Geometry check sheet. Reference: the model listing, model coordinates, mm. Face numbers are marked on the shaded views. A direction names the side the tool comes from. Round coordinates to 2 decimals unless told otherwise and drop trailing zeros. Write each loop counter-clockwise with the first axis right and the second up, starting at its lowest first coordinate (ties: lowest second). Pieces come first, ordered by that corner, then holes. Notation, with made-up numbers: (-7.5, 19.5) -> (25.5, 19.5) arc R22 ccw to (25.5, 46.5) -> close; hole circle Ø2 at (-33.75, 49.25). An arc over 180 degrees is marked (long way). Use a Markdown table: item, result.
```python
from build123d import *

# Parameters (mm, degrees)
BOSS_EXTRUDE1_DEPTH = 12
SKETCH2_R           = 17.5
BOSS_EXTRUDE2_DEPTH = 1
SKETCH3_R           = 0.75
BOSS_EXTRUDE3_DEPTH = 5
FILLET1_R           = 1.5
CUT_EXTRUDE6_REACH  = 67.15
SKETCH6_R           = 2.85
CHAMFER1_SIZE       = 0.5


with BuildPart() as part:
    # Sketch1 → Boss-Extrude1 (new body)
    with BuildSketch(Plane(origin=(0, 0, 0), x_dir=(1, 0, 0), z_dir=(0, 1, 0))):
        with BuildLine():
            Line((-28.55, 22.55), (-28.55, -22.55))
            ThreePointArc((-28.55, -22.55), (-26.792640687, -26.792640687), (-22.55, -28.55))
            Line((-22.55, -28.55), (22.55, -28.55))
            ThreePointArc((22.55, -28.55), (26.792640687, -26.792640687), (28.55, -22.55))
            Line((28.55, -22.55), (28.55, 22.55))
            ThreePointArc((28.55, 22.55), (26.792640687, 26.792640687), (22.55, 28.55))
            Line((22.55, 28.55), (-22.55, 28.55))
            ThreePointArc((-22.55, 28.55), (-26.792640687, 26.792640687), (-28.55, 22.55))
        make_face()
        with BuildLine():
            Line((-22.55, 27.55), (22.55, 27.55))
            ThreePointArc((22.55, 27.55), (26.085533906, 26.085533906), (27.55, 22.55))
            Line((27.55, 22.55), (27.55, -22.55))
            ThreePointArc((27.55, -22.55), (26.085533906, -26.085533906), (22.55, -27.55))
            Line((22.55, -27.55), (-22.55, -27.55))
            ThreePointArc((-22.55, -27.55), (-26.085533906, -26.085533906), (-27.55, -22.55))
            Line((-27.55, -22.55), (-27.55, 22.55))
            ThreePointArc((-27.55, 22.55), (-26.085533906, 26.085533906), (-22.55, 27.55))
        make_face(mode=Mode.SUBTRACT)
    extrude(amount=BOSS_EXTRUDE1_DEPTH)

    # Sketch2 → Boss-Extrude2 (add)
    with BuildSketch(Plane(origin=(0, 12, 0), x_dir=(1, 0, 0), z_dir=(0, 1, 0))):
        with BuildLine():
            Line((-22.55, -28.55), (22.55, -28.55))
            ThreePointArc((22.55, -28.55), (26.792640687, -26.792640687), (28.55, -22.55))
            Line((28.55, -22.55), (28.55, 22.55))
            ThreePointArc((28.55, 22.55), (26.792640687, 26.792640687), (22.55, 28.55))
            Line((22.55, 28.55), (-22.55, 28.55))
            ThreePointArc((-22.55, 28.55), (-26.792640687, 26.792640687), (-28.55, 22.55))
            Line((-28.55, 22.55), (-28.55, -22.55))
            ThreePointArc((-28.55, -22.55), (-26.792640687, -26.792640687), (-22.55, -28.55))
        make_face()
        with Locations(Location((0, 0, 0), (0, 0, 270))):
            Circle(SKETCH2_R, mode=Mode.SUBTRACT)
    extrude(amount=BOSS_EXTRUDE2_DEPTH)

    # Sketch3 → Boss-Extrude3 (add, symmetric)
    with BuildSketch(Plane.ZY):
        with Locations((-27.55, 0.75)):
            Circle(SKETCH3_R)
        with Locations((27.55, 0.75)):
            Circle(SKETCH3_R)
    extrude(amount=BOSS_EXTRUDE3_DEPTH, both=True)

    # Fillet1
    fillet1_edges = [part.edges().sort_by_distance(p)[0] for p in [
        (-26.792640687, 13, 26.792640687),
        (0, 13, 28.55),
        (26.792640687, 13, 26.792640687),
        (28.55, 13, 0),
        (26.792640687, 13, -26.792640687),
        (0, 13, -28.55),
        (-26.792640687, 13, -26.792640687),
        (-28.55, 13, 0),
    ]]
    fillet(fillet1_edges, radius=FILLET1_R)

    # Sketch6 → Cut-Extrude6 (cut, up to next)
    with BuildSketch(Plane.ZY.offset(28.55), mode=Mode.PRIVATE) as cut_extrude6_sk1:
        with Locations((-12.78, 7.73)):
            Circle(SKETCH6_R)
    cut_extrude6_tool1 = extrude(cut_extrude6_sk1.sketch, amount=-CUT_EXTRUDE6_REACH, mode=Mode.PRIVATE) & part.part
    # Sketch6 → Cut-Extrude6 (cut, up to next)
    with BuildSketch(Plane.ZY.offset(28.55), mode=Mode.PRIVATE) as cut_extrude6_sk2:
        with BuildLine():
            Line((-3.19, 3.82), (3.189999856, 3.82))
            ThreePointArc((3.189999856, 3.82), (4.236517943, 4.253481955), (4.67, 5.3))
            Line((4.67, 5.3), (4.67, 5.9))
            ThreePointArc((4.67, 5.9), (4.236518036, 6.946518036), (3.19, 7.38))
            Line((3.19, 7.38), (-3.19, 7.38))
            ThreePointArc((-3.19, 7.38), (-4.236518036, 6.946518036), (-4.67, 5.9))
            Line((-4.67, 5.9), (-4.67, 5.3))
            ThreePointArc((-4.67, 5.3), (-4.236518036, 4.253481964), (-3.19, 3.82))
        make_face()
    cut_extrude6_tool2 = extrude(cut_extrude6_sk2.sketch, amount=-CUT_EXTRUDE6_REACH, mode=Mode.PRIVATE) & part.part
    add(cut_extrude6_tool1.solids().sort_by_distance((-28.55, 7.73, -12.78))[0], mode=Mode.SUBTRACT)
    add(cut_extrude6_tool2.solids().sort_by_distance((-28.55, 5.6, 0))[0], mode=Mode.SUBTRACT)

    # Chamfer1
    chamfer1_edges = [part.edges().sort_by_distance(p)[0] for p in [
        (-28.55, 4.253481964, -4.236518036),
        (-28.55, 3.82, -7.2e-08),
        (-28.55, 4.253481955, 4.236517943),
        (-28.55, 5.6, 4.67),
        (-28.55, 6.946518036, 4.236518036),
        (-28.55, 7.38, 0),
        (-28.55, 6.946518036, -4.236518036),
        (-28.55, 5.6, -4.67),
        (-28.55, 7.73, -15.63),
    ]]
    chamfer(chamfer1_edges, length=CHAMFER1_SIZE)


solid = part.part
```
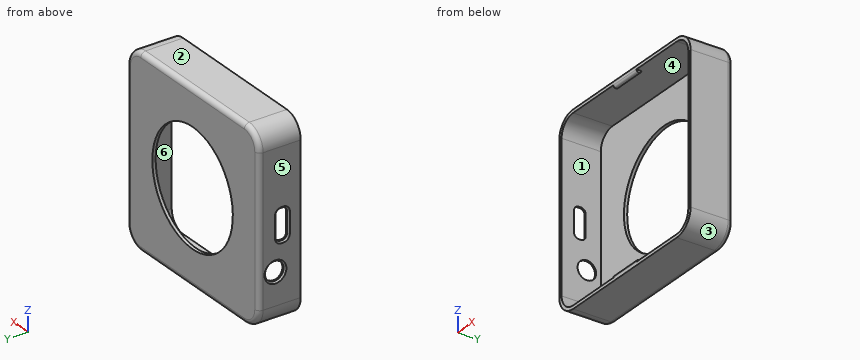
(1) Access from +Z, -Z, +X, -X, +Y, -Y to the whole of each face (thin tool, end or side, straight path). Record for the marked faces 4, 5 and 6.
A:
| item | result |
|---|---|
| face 4 | none |
| face 5 | +Z, -Z, -X, +Y, -Y |
| face 6 | -Y |
(2) Section check D-D on x = -6. Record the cut outline in (y, z), plus the area to 3 significant figures.
A:
| item | result |
|---|---|
| outline | (0, -28.55) -> (11.5, -28.55) arc R1.5 ccw to (13, -27.05) -> (13, -16.44) -> (12, -16.44) -> (12, -27.55) -> (0, -27.55) -> close; (0, 27.55) -> (12, 27.55) -> (12, 16.44) -> (13, 16.44) -> (13, 27.05) arc R1.5 ccw to (11.5, 28.55) -> (0, 28.55) -> close |
| area | 47.3 mm2 |
(3) Release check for a two-part mould opening along Z. For the marked faces 1, 2 and 3 record: +Z half, -Z half, draft (parallel to the pull), parting line (faces both ways), or undercut.
A:
| item | result |
|---|---|
| face 1 | undercut |
| face 2 | +Z half |
| face 3 | -Z half |
(4) Section check C-C on y = 0.75. Record the cut outline in (x, z), plus the area to 3 significant figures.
A:
| item | result |
|---|---|
| outline | (-28.55, -22.55) arc R6 ccw to (-22.55, -28.55) -> (22.55, -28.55) arc R6 ccw to (28.55, -22.55) -> (28.55, 22.55) arc R6 ccw to (22.55, 28.55) -> (-22.55, 28.55) arc R6 ccw to (-28.55, 22.55) -> close; hole (-27.55, -22.55) arc R5 ccw to (-22.55, -27.55) -> (-5, -27.55) -> (-5, -26.8) -> (5, -26.8) -> (5, -27.55) -> (22.55, -27.55) arc R5 ccw to (27.55, -22.55) -> (27.55, 22.55) arc R5 ccw to (22.55, 27.55) -> (5, 27.55) -> (5, 26.8) -> (-5, 26.8) -> (-5, 27.55) -> (-22.55, 27.55) arc R5 ccw to (-27.55, 22.55) -> close |
| area | 230 mm2 |
(5) Section check B-B on z = 0. Record the cut outline in (x, y), plus the area to 3 significant figures.
A:
| item | result |
|---|---|
| outline | (-28.55, 0) -> (-27.55, 0) -> (-27.55, 3.82) -> (-28.05, 3.82) -> (-28.55, 3.32) -> close; (-28.55, 7.88) -> (-28.05, 7.38) -> (-27.55, 7.38) -> (-27.55, 12) -> (-17.5, 12) -> (-17.5, 13) -> (-27.05, 13) arc R1.5 ccw to (-28.55, 11.5) -> close; (17.5, 12) -> (27.55, 12) -> (27.55, 0) -> (28.55, 0) -> (28.55, 11.5) arc R1.5 ccw to (27.05, 13) -> (17.5, 13) -> close |
| area | 41.3 mm2 |
(6) Thickness scan on line 1 (Z direction, x = -15, y = 2.75); line 2 (X direction, y = 12.25, z = 0). Record the ranges inside material, lowest first.
A:
| item | result |
|---|---|
| line 1 | z = -28.55 to -27.55, 27.55 to 28.55 |
| line 2 | x = -28.35 to -17.5, 17.5 to 28.35 |
(7) Gauge pin test, flat ends, axial feed: pin 1 Ø0.6 at (y, z) = (1, -27.5) entering from -X; pin 2 Ø16.5 at (x, z) = (-12, -9) entering from -Y; pin 3 Ø0.6 at (x, y) = (-28, 5.5) entering from -Z. Record the tip position at first contact, or that the pin passes through.
A:
| item | result |
|---|---|
| pin 1 | stops at x = -26.34 |
| pin 2 | stops at y = 12 |
| pin 3 | stops at z = -25.63 |
(8) Section check A-A on x = 14. Record the cut outline in (y, z).
A:
| item | result |
|---|---|
| outline | (0, -28.55) -> (11.5, -28.55) arc R1.5 ccw to (13, -27.05) -> (13, -10.5) -> (12, -10.5) -> (12, -27.55) -> (0, -27.55) -> close; (0, 27.55) -> (12, 27.55) -> (12, 10.5) -> (13, 10.5) -> (13, 27.05) arc R1.5 ccw to (11.5, 28.55) -> (0, 28.55) -> close |
